The model under review builds one solid part; all positions refer to its coordinate system, in mm. Face numbers are marked on the shaded views. Round coordinates to 2 decimals unless told otherwise and drop trailing zeros. Order: outer loops, then holes, each group sorted by start corner. A loop starts at its lowest first (then second) coordinate and runs counter-clockwise, first axis right, second up. Notation, with made-up numbers: M 49,-8 L 61,-8 A30 cw 61,22 Z; hole C 64,25 d11. An arc over 180 degrees is marked long. Answer as a JSON object with one key per item and string values. Group by question number.
1. Add section C-C on x = -12.5. State the section outline as (y, z) points (1 decimal), and give its area (3 significant figures).
2. To check wall thickness, follow probe 1 along Z at (x, y) = (-12.5, 0); probe 2 along Y at (x, z) = (-5.25, 0). State the ranges of each line that lie inside material, in increasing order. Write a range as [from, to].
3. Add section D-D on x = -17.5. State the section outline as (y, z) points (1 decimal), and give its area (3 significant figures).
4. Mouldability with a two-part tool opening along Y and no side actions: class the marked faces 1, 2 and 3 as released by +Y, released by -Y, zero draft, split by the parting line, or undercut.
5. Clearance check with flat-ended pins moving along their axes: P1, Ø8, axis at x = -9.5, y = -5, coming from the -Z side; P2, Ø4, axis at x = -6, z = 9.5, coming from the -Y side; P3, Ø10, axis at x = -11.5, y = 4, coming from the -Z side. State where each tip first meets the part, or that it passes through.
6. Add section A-A on y = 0. State the section outline as (x, z) points (1 decimal).
```python
from build123d import *


with BuildPart() as part:
    # Sketch1 → Base-Revolve (revolve)
    with BuildSketch(Plane.XY):
        with BuildLine():
            Line((0, 12.125), (0, 16.5))
            ThreePointArc((0, 16.5), (-0.146446609, 16.853553391), (-0.5, 17))
            Line((-0.5, 17), (-10.5, 17))
            ThreePointArc((-10.5, 17), (-10.853553391, 17.146446609), (-11, 17.5))
            Line((-11, 17.5), (-11, 19.5))
            ThreePointArc((-11, 19.5), (-11.146446609, 19.853553391), (-11.5, 20))
            Line((-11.5, 20), (-17, 20))
            ThreePointArc((-17, 20), (-18.414213562, 19.414213562), (-19, 18))
            Line((-19, 18), (-19, 12.125))
            Line((-19, 12.125), (-18.30284955, 10.9175))
            Line((-18.30284955, 10.9175), (-0.69715045, 10.9175))
            Line((-0.69715045, 10.9175), (0, 12.125))
        make_face()
    revolve(axis=Axis((0, 0, 0), (-1, 0, 0)))


solid = part.part
```
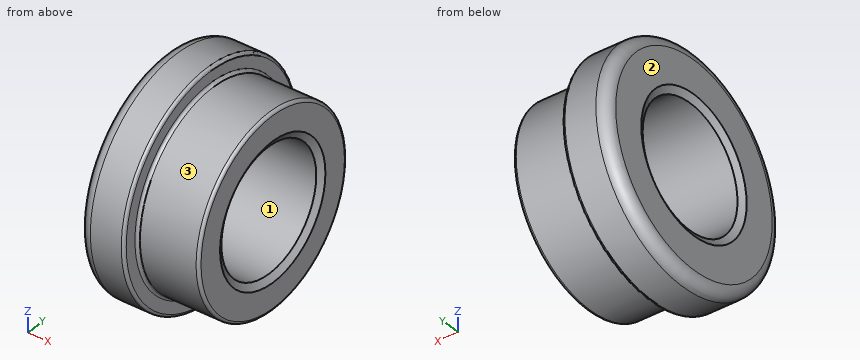
Recorded:
{
 "1": {"outline": "C 0,0 d40; hole C 0,0 d21.8", "area": "882 mm²"},
 "2": {"probe 1": "z = [-20, -10.92], [10.92, 20]", "probe 2": "y = [-17, -10.92], [10.92, 17]"},
 "3": {"outline": "C 0,0 d39.9; hole C 0,0 d21.8", "area": "874 mm²"},
 "4": {"face 1": "undercut", "face 2": "zero draft", "face 3": "split by the parting line"},
 "5": {"P1": "stops at z = -19.94", "P2": "stops at y = -15.26", "P3": "stops at z = -20"},
 "6": {"outline": "M -19,-18 A2 ccw -17,-20 L -11.5,-20 A0.5 ccw -11,-19.5 L -11,-17.5 A0.5 cw -10.5,-17 L -0.5,-17 A0.5 ccw 0,-16.5 L 0,-12.1 L -0.7,-10.9 L -18.3,-10.9 L -19,-12.1 Z; M -19,12.1 L -18.3,10.9 L -0.7,10.9 L 0,12.1 L 0,16.5 A0.5 ccw -0.5,17 L -10.5,17 A0.5 cw -11,17.5 L -11,19.5 A0.5 ccw -11.5,20 L -17,20 A2 ccw -19,18 Z"}
}
